Design review of the part built by this model. Coordinates are the model's own, in mm. Face numbers are marked on the shaded views. A direction names the side the tool comes from. Give positions to 0.01 mm unless a question says otherwise; leave off trailing zeros. Loops run counter-clockwise (first coordinate to the right, second up) from the corner with the lowest first, then second, coordinate; pieces in that order, holes last. Notation, with made-up numbers: (56, -27) -> (109, -27) arc R25 cw to (109, -5) -> close; hole circle Ø8 at (42.5, 24). An arc over 180 degrees is marked (long way). Use a Markdown table: item, result. Add a question column.
1. Add section C-C (x = -59). State the section outline as (y, z) points.
2. Add section B-B (x = 0). State the section outline as (y, z) points.
3. Add section A-A (z = -70). State the section outline as (x, y) points.
4. To check wall thickness, follow line 1 (X direction, y = -97, z = -73); line 2 (Y direction, x = 0, z = -80.5); line 3 (Y direction, x = 0, z = -59). State the ranges of each line that lie inside material, in increasing order.
5. Draft analysis for pull direction Z (two halves, no side actions). For the marked faces 1, 2, 3 and 4, state which applies: pulls with the +Z half, pulls with the -Z half, needs draft (parallel to the pull), parting line crosses it, or undercut.
6. For pin 1 Ø12 at (y, z) = (-68, -66) entering from +X; pin 2 Ø3 at (x, y) = (-28.5, -23.5) entering from +Z; pin 3 Ø10 at (x, z) = (-19.5, -21) entering from -Y, all flat-tipped, find the tip position at first contact; note any pin that passes through.
7. Add section D-D (z = -16.5). State the section outline as (x, y) points.
8. For the marked faces 5, 6, 7, 8 and 9, list the 3-axis set-ups (+Z, -Z, +X, -X, +Y, -Y) from which the entire face can be reached by the end or side of a thin tool; tool diameter is ignored.
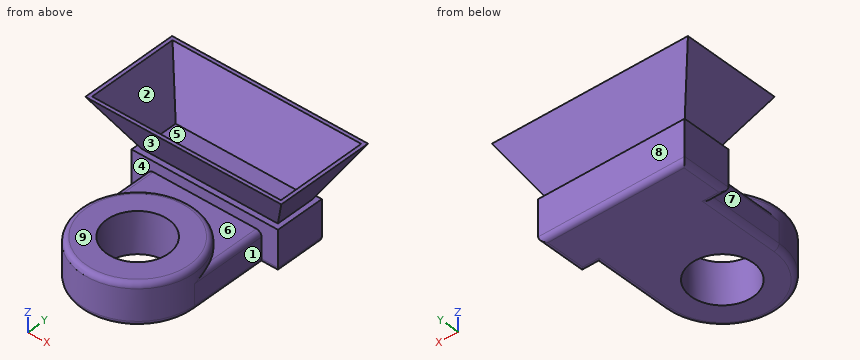
```python
from build123d import *

# Parameters (mm, degrees)
LIGHT_PROFILE_W               = 190
LIGHT_PROFILE_H               = 95
LIGHT_EXTRUDE_DEPTH           = 50
LIGHT_EXTRUDE_DRAFT           = -30
LIGHT_SHELL_T                 = -3
ELECTRONICS_BOX_SKETCH_W      = 142
ELECTRONICS_BOX_SKETCH_H      = 48
ELECTRONICS_BOX_EXTRUDE_DEPTH = 40
SUPPORT_EXTRUDE_DEPTH         = 40
BACK_FILLET_R                 = 5
WRIST_HOLE_SKETCH_R           = 30
WRIST_HOLE_CUT_DEPTH          = 40
SUPPORT_INSET_CUT_DEPTH       = 10
FRONT_FILLET_R                = 5


with BuildPart() as part:
    # Light Profile → Light Extrude (with draft: the straight prism first)
    with BuildSketch(Plane.XY):
        Rectangle(LIGHT_PROFILE_W, LIGHT_PROFILE_H)
    extrude(amount=-LIGHT_EXTRUDE_DEPTH)
    # Light Extrude: the draft: its side faces are tilted about the plane it starts from
    light_extrude_sides = [part.faces().sort_by_distance(p)[0] for p in [
        (-95, 0, -25),
        (0, -47.5, -25),
        (95, 0, -25),
        (0, 47.5, -25),
    ]]
    draft(light_extrude_sides, Plane.XY, LIGHT_EXTRUDE_DRAFT)

    # Light Shell
    light_shell_openings = [part.faces().sort_by_distance(p)[0] for p in [
        (0, 0, 0),
    ]]
    offset(amount=LIGHT_SHELL_T, openings=light_shell_openings, kind=Kind.INTERSECTION)

    # Electronics Box Sketch → Electronics Box Extrude (add)
    with BuildSketch(Plane(origin=(0, 0, -50), x_dir=(-1, 0, 0), z_dir=(0, 0, -1))):
        Rectangle(ELECTRONICS_BOX_SKETCH_W, ELECTRONICS_BOX_SKETCH_H)
    extrude(amount=ELECTRONICS_BOX_EXTRUDE_DEPTH)

    # Support Sketch → Support Extrude (add)
    with BuildSketch(Plane.XY.offset(-50)):
        with BuildLine():
            Line((55, -97.5), (55, -24))
            Line((55, -24), (-55, -24))
            Line((-55, -24), (-55, -97.5))
            ThreePointArc((-55, -97.5), (0, -152.5), (55, -97.5))
        make_face()
    extrude(amount=-SUPPORT_EXTRUDE_DEPTH)

    # Back Fillet
    back_fillet_edges = [part.edges().sort_by_distance(p)[0] for p in [
        (-71, 0, -90),
        (0, 24, -90),
        (71, 0, -90),
        (63, -24, -90),
        (-63, -24, -90),
        (55, -60.75, -90),
        (-55, -60.75, -90),
        (0, -152.5, -90),
    ]]
    fillet(back_fillet_edges, radius=BACK_FILLET_R)

    # Wrist Hole Sketch → Wrist Hole Cut (cut)
    with BuildSketch(Plane(origin=(0, 0, -90), x_dir=(-1, 0, 0), z_dir=(0, 0, -1))):
        with Locations((0, -97.5)):
            Circle(WRIST_HOLE_SKETCH_R)
    extrude(amount=-WRIST_HOLE_CUT_DEPTH, mode=Mode.SUBTRACT)

    # Support Inset Sketch → Support Inset Cut (cut)
    with BuildSketch(Plane.XY.offset(-50)):
        with BuildLine():
            Line((-55, -24), (55, -24))
            Line((55, -24), (55, -42.5))
            Line((55, -42.5), (55, -97.5))
            ThreePointArc((55, -97.5), (0, -42.5), (-55, -97.5))
            Line((-55, -97.5), (-55, -42.5))
            Line((-55, -42.5), (-55, -24))
        make_face()
    extrude(amount=-SUPPORT_INSET_CUT_DEPTH, mode=Mode.SUBTRACT)

    # Front Fillet
    # the kernel refuses this fillet: 5 mm, written as the material it takes off along each edge
    with BuildSketch(Plane(origin=(0, -97.5, -50), x_dir=(-1, 0, 0), z_dir=(0, -1, 0))) as front_fillet_piece_1:
        with BuildLine():
            CenterArc((55 - FRONT_FILLET_R, FRONT_FILLET_R), FRONT_FILLET_R, 270, 90)
            Line((55, FRONT_FILLET_R), (55, 0))
            Line((55, 0), (55 - FRONT_FILLET_R, 0))
        make_face()
    revolve(axis=Axis((0, -97.5, -50), (0, 0, -1)), mode=Mode.SUBTRACT)
    with BuildSketch(Plane(origin=(-55, -24, -60), x_dir=(1, 0, 0), z_dir=(0, -1, 0))) as front_fillet_piece_2_section:
        with BuildLine():
            CenterArc((FRONT_FILLET_R, -FRONT_FILLET_R), FRONT_FILLET_R, 90, 90)
            Line((0, -FRONT_FILLET_R), (0, 0))
            Line((0, 0), (FRONT_FILLET_R, 0))
        make_face()
    front_fillet_piece_2 = extrude(amount=86, mode=Mode.PRIVATE)
    front_fillet_piece_2 = front_fillet_piece_2 - Plane(origin=(0, -97.5, -61.160200813), x_dir=(-1, 0, 0), z_dir=(0, 0, 1)) * Cylinder(55, 192, mode=Mode.PRIVATE)
    add(front_fillet_piece_2, mode=Mode.SUBTRACT)
    with BuildSketch(Plane(origin=(55, -110, -60), x_dir=(0, 0, -1), z_dir=(0, 1, 0))) as front_fillet_piece_3_section:
        with BuildLine():
            CenterArc((FRONT_FILLET_R, FRONT_FILLET_R), FRONT_FILLET_R, 180, 90)
            Line((0, FRONT_FILLET_R), (0, 0))
            Line((0, 0), (FRONT_FILLET_R, 0))
        make_face()
    front_fillet_piece_3 = extrude(amount=86, mode=Mode.PRIVATE)
    front_fillet_piece_3 = front_fillet_piece_3 - Plane(origin=(0, -97.5, -61.160225753), x_dir=(-1, 0, 0), z_dir=(0, 0, 1)) * Cylinder(55, 192, mode=Mode.PRIVATE)
    add(front_fillet_piece_3, mode=Mode.SUBTRACT)


solid = part.part
```
Taken from the geometry:
| question | item | result |
|---|---|---|
| 1 | outline | (-47.5, 0) -> (-18.63, -50) -> (-24, -50) -> (-24, -85) arc R5 ccw to (-19, -90) -> (19, -90) arc R5 ccw to (24, -85) -> (24, -50) -> (18.63, -50) -> (47.5, 0) -> (44.04, 0) -> (16.9, -47) -> (-16.9, -47) -> (-44.04, 0) -> close |
| 2 | outline | (-152.5, -85) arc R5 ccw to (-147.5, -90) -> (-127.5, -90) -> (-127.5, -50) -> (-147.5, -50) arc R5 ccw to (-152.5, -55) -> close; (-67.5, -90) -> (19, -90) arc R5 ccw to (24, -85) -> (24, -50) -> (18.63, -50) -> (47.5, 0) -> (44.04, 0) -> (16.9, -47) -> (-16.9, -47) -> (-44.04, 0) -> (-47.5, 0) -> (-18.63, -50) -> (-24, -50) -> (-24, -60) -> (-42.5, -60) -> (-42.5, -55) arc R5 ccw to (-47.5, -50) -> (-67.5, -50) -> close |
| 3 | outline | (-71, -24) -> (-55, -24) -> (-55, -97.5) arc R55 ccw to (55, -97.5) -> (55, -24) -> (71, -24) -> (71, 24) -> (-71, 24) -> close; hole circle Ø60 at (0, -97.5) |
| 4 | line 1 | x = -55 to -30, 30 to 55 |
| 4 | line 2 | y = -152.5 to -127.5, -67.5 to 24 |
| 4 | line 3 | y = -152.5 to -127.5, -67.5 to -42.5, -24 to 24 |
| 5 | face 1 | needs draft |
| 5 | face 2 | pulls with the +Z half |
| 5 | face 3 | undercut |
| 5 | face 4 | undercut |
| 6 | pin 1 | stops at x = 55 |
| 6 | pin 2 | stops at z = -32.97 |
| 6 | pin 3 | stops at y = -38.26 |
| 7 | outline | (-85.47, -37.97) -> (85.47, -37.97) -> (85.47, 37.97) -> (-85.47, 37.97) -> close; hole (-82.01, -34.51) -> (82.01, -34.51) -> (82.01, 34.51) -> (-82.01, 34.51) -> close |
| 8 | face 5 | +Z |
| 8 | face 6 | none |
| 8 | face 7 | -Z, -X, -Y |
| 8 | face 8 | -Z, +X, -X, +Y |
| 8 | face 9 | +Z, +X, -X, -Y |
